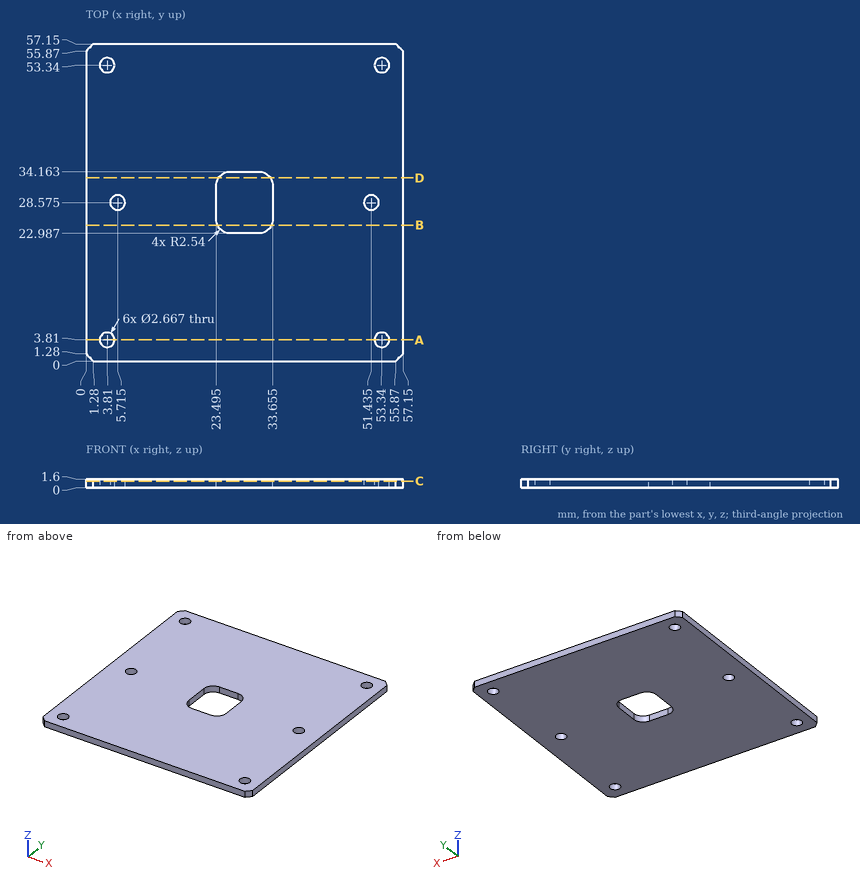
Check sheet for the drawn part. Datum: minimum x, y, z corner. Units: mm. Round coordinates to 2 decimals unless told otherwise and drop trailing zeros. Order: outer loops, then holes, each group sorted by start corner. A loop starts at its lowest first (then second) coordinate and runs counter-clockwise, first axis right, second up. Notation, with made-up numbers: (84.25, 21.5) -> (140.25, 21.5) arc R26 ccw to (140.25, 35.5) -> close; hole circle Ø5 at (13.25, 40). An arc over 180 degrees is marked (long way). Put each result on its own line as item: value.
1) Section check C-C (z = 1.2). Give the number of separate pieces and of enclosed holes in the cut face, then the cut area to 3 significant figures.
Final values:
separate pieces: 1
enclosed holes: 7
area: 3,120 mm^2
2) Material ranges on line 1 (X direction, y = 53.34, z = 0.5); line 2 (Y direction, x = 24.5, z = 0.35), recorded low to high.
Final values:
line 1: x = 0 to 2.48, 5.14 to 52.01, 54.67 to 57.15
line 2: y = 0 to 23.5, 33.65 to 57.15
3) Section check B-B (y = 24.5). Record the cut outline in (x, z).
Final values:
outline: (0, 0) -> (23.71, 0) -> (23.71, 1.6) -> (0, 1.6) -> close; (33.44, 0) -> (57.15, 0) -> (57.15, 1.6) -> (33.44, 1.6) -> close
4) Section check D-D (y = 33). Record the cut outline in (x, z).
Final values:
outline: (0, 0) -> (23.9, 0) -> (23.9, 1.6) -> (0, 1.6) -> close; (33.25, 0) -> (57.15, 0) -> (57.15, 1.6) -> (33.25, 1.6) -> close
5) Section check A-A (y = 3.81). Record the cut outline in (x, z), then the cut area to 3 significant figures.
Final values:
outline: (0, 0) -> (2.48, 0) -> (2.48, 1.6) -> (0, 1.6) -> close; (5.14, 0) -> (52.01, 0) -> (52.01, 1.6) -> (5.14, 1.6) -> close; (54.67, 0) -> (57.15, 0) -> (57.15, 1.6) -> (54.67, 1.6) -> close
area: 82.9 mm^2
6) Depth check by flat-ended pin: pin 1 (2.5 mm diameter, centred on x = 53.34, y = 3.81, fed in from -Z). Enter the tip coordinate at first touch or a pass-through.
Final values:
pin 1: passes through
